```python
from build123d import *

# Parameters (mm, degrees)
SKETCH1_W           = 21
SKETCH1_H           = 1.747373259
SKETCH1_H_2         = 0.25
SKETCH1_W_2         = 23
SKETCH1_H_3         = 49.505253482
SKETCH1_W_3         = 17.25
BOSS_EXTRUDE1_DEPTH = 1
SKETCH2_W           = 23
SKETCH2_H           = 1.5
SKETCH2_W_2         = 2.5
SKETCH2_W_3         = 8
BOSS_EXTRUDE2_DEPTH = 5
SKETCH3_W           = 2.5
SKETCH3_H           = 1.5
BOSS_EXTRUDE3_DEPTH = 2
SKETCH4_W           = 3
SKETCH4_H           = 1.997373259
SKETCH4_W_2         = 10
BOSS_EXTRUDE4_DEPTH = 11
SKETCH5_W           = 4
SKETCH5_H           = 2.002626741
BOSS_EXTRUDE5_DEPTH = 7
FILLET1_R           = 1


with BuildPart() as part:
    # Sketch1 → Boss-Extrude1 (new body)
    with BuildSketch(Plane.XY):
        with Locations((0, 25.876313371)):
            Rectangle(SKETCH1_W, SKETCH1_H)
        with Locations((0, 24.877626741)):
            Rectangle(SKETCH1_W, SKETCH1_H_2)
        Rectangle(SKETCH1_W_2, SKETCH1_H_3)
        with Locations((0.875, -24.877626741)):
            Rectangle(SKETCH1_W_3, SKETCH1_H_2)
        with Locations((0.875, -25.876313371)):
            Rectangle(SKETCH1_W_3, SKETCH1_H)
    extrude(amount=-BOSS_EXTRUDE1_DEPTH)

    # Sketch2 → Boss-Extrude2 (add)
    with BuildSketch(Plane(origin=(0, 0, -1), x_dir=(-1, 0, 0), z_dir=(0, 0, -1))):
        with Locations((0, -19.002626741)):
            Rectangle(SKETCH2_W, SKETCH2_H)
        with Locations((-10.25, 8.502626741)):
            Rectangle(SKETCH2_W_2, SKETCH2_H)
        with Locations((0, 8.502626741)):
            Rectangle(SKETCH2_W_3, SKETCH2_H)
        with Locations((10.25, 8.502626741)):
            Rectangle(SKETCH2_W_2, SKETCH2_H)
    extrude(amount=BOSS_EXTRUDE2_DEPTH)

    # Sketch3 → Boss-Extrude3 (add)
    with BuildSketch(Plane(origin=(0, 0, -6), x_dir=(-1, 0, 0), z_dir=(0, 0, -1))):
        with Locations((-10.25, 8.502626741)):
            Rectangle(SKETCH3_W, SKETCH3_H)
        with Locations((10.25, 8.502626741)):
            Rectangle(SKETCH3_W, SKETCH3_H)
        with Locations((-10.25, -19.002626741)):
            Rectangle(SKETCH3_W, SKETCH3_H)
        with Locations((10.25, -19.002626741)):
            Rectangle(SKETCH3_W, SKETCH3_H)
    extrude(amount=BOSS_EXTRUDE3_DEPTH)

    # Sketch4 → Boss-Extrude4 (add)
    with BuildSketch(Plane(origin=(0, 0, -1), x_dir=(-1, 0, 0), z_dir=(0, 0, -1))):
        with Locations((-9, 25.751313371)):
            Rectangle(SKETCH4_W, SKETCH4_H)
        with Locations((5.5, 25.751313371)):
            Rectangle(SKETCH4_W_2, SKETCH4_H)
    extrude(amount=BOSS_EXTRUDE4_DEPTH)

    # Sketch5 → Boss-Extrude5 (add)
    with BuildSketch(Plane(origin=(0, 0, -1), x_dir=(-1, 0, 0), z_dir=(0, 0, -1))):
        with Locations((9.5, 23.751313371)):
            Rectangle(SKETCH5_W, SKETCH5_H)
        Polygon((8, -24.752626741), (11.5, -24.752626741), (11.5, -19.752626741), (9, -19.752626741), (9, -21.75), (8, -21.75), align=None)
        Polygon((-11.5, -24.752626741), (-8, -24.752626741), (-8, -21.75), (-9, -21.75), (-9, -19.752626741), (-11.5, -19.752626741), align=None)
    extrude(amount=BOSS_EXTRUDE5_DEPTH)

    # Fillet1
    fillet1_edges = [part.edges().sort_by_distance(p)[0] for p in [
        (7.5, 25.75131337, -1),
        (-0.5, 25.75131337, -1),
        (-4, 8.502626741, -1),
        (4, 8.502626741, -1),
        (9, 8.502626741, -1),
        (-9, 8.502626741, -1),
    ]]
    fillet(fillet1_edges, radius=FILLET1_R)


solid = part.part
```
Can you work these out from the model? Positions are in its coordinate system, mm. A direction names the side the tool comes from. Round coordinates to 2 decimals unless told otherwise and drop trailing zeros. Loops run counter-clockwise (first coordinate to the right, second up) from the corner with the lowest first, then second, coordinate; pieces in that order, holes last. Notation, with made-up numbers: M 4,-12.75 L 28,-12.75 A23 cw 28,14.25 Z; hole C 78.25,-8 d6. An arc over 180 degrees is marked long. Answer in a Markdown table with one row per item.
1. Please list where these lines run through material, in increasing order: line 1 (Y direction, x = -9.5, z = -5.5); line 2 (Y direction, x = 8.25, z = -3.25); line 3 (Y direction, x = 0.75, z = -5). Write a range as from..to.
Established:
| item | result |
|---|---|
| line 1 | -24.75..-18.25, 7.75..9.25, 22.75..26.75 |
| line 2 | -24.75..-21.75, -19.75..-18.25, 24.75..26.75 |
| line 3 | -19.75..-18.25, 7.75..9.25 |
2. I'm going to push flat-ended pins straight in: pin 1 Ø1 at (x, z) = (9.5, -4.5) entering from -Y; pin 2 Ø4 at (x, z) = (-3.5, -4) entering from -Y; pin 3 Ø5 at (x, y) = (3.5, -5.5) entering from -Z. Where does each tip first touch, or does it pass through?
Established:
| item | result |
|---|---|
| pin 1 | y = -24.75 |
| pin 2 | y = -19.75 |
| pin 3 | z = -1 |
3. If we section it at A-A, the plane z = -10.5: Please give me the cut outline in (x, y), plus the area to 3 significant figures.
Established:
| item | result |
|---|---|
| outline | M -10.5,24.75 L -0.5,24.75 L -0.5,26.75 L -10.5,26.75 Z; M 7.5,24.75 L 10.5,24.75 L 10.5,26.75 L 7.5,26.75 Z |
| area | 26.0 mm² |
4. Thinking about a two-plate mould opening in Y: for faces 1 (the face through (9.5, -25.8, -0.5)), 2 (the face through (-8.715, 8.513, -1.301)), 3 (the face through (-10, -24.753, -4)), 4 (the face through (9, 24.753, -6)), which applies, pulls with the +Y half, pulls with the -Y half, needs draft (parallel to the pull), parting line crosses it, or undercut?
Established:
| item | result |
|---|---|
| face 1 | needs draft |
| face 2 | undercut |
| face 3 | pulls with the -Y half |
| face 4 | undercut |
5. On a 3-axis mill with a long thin cutter (end or side, diameter ignored), from which of +Z, -Z, +X, -X, +Y, -Y can I reach the whole of each face in a straight line? I mean faces 5 (the face through (-9, -20, -5)), 6 (the face through (-8, -23, -4)), 7 (the face through (7.5, 26, -7)), 8 (the face through (-10, -21, -8)). Say none if no direction works.
Established:
| item | result |
|---|---|
| face 5 | -Z |
| face 6 | -Z, -Y |
| face 7 | -Z, +Y |
| face 8 | -Z, +X, -X, -Y |
6. If we section it at C-C, the plane x = -6.25: Please give me the cut outline in (y, z), plus the area to 3 significant figures.
Established:
| item | result |
|---|---|
| outline | M -26.75,-1 L -19.75,-1 L -19.75,-6 L -18.25,-6 L -18.25,-1 L 24.75,-1 L 24.75,-12 L 26.75,-12 L 26.75,0 L -26.75,0 Z |
| area | 83.0 mm² |
7. If we section it at B-B, the plane z = -7: Give the number of separate pieces and of enclosed holes in the cut face, plus the area to 3 significant figures.
Established:
| item | result |
|---|---|
| separate pieces | 6 |
| enclosed holes | 0 |
| area | 80.0 mm² |
8. If we section it at D-D, the plane y = 23.5: Please give me the cut outline in (x, z), plus the area to 3 significant figures.
Established:
| item | result |
|---|---|
| outline | M -11.5,-8 L -7.5,-8 L -7.5,-1 L 11.5,-1 L 11.5,0 L -11.5,0 Z |
| area | 51.0 mm² |
